from build123d import *

# Parameters (mm, degrees)
BOSS_EXTRUDE1_DEPTH = 63.5
SKETCH3_W           = 52.197
SKETCH3_H           = 52.197
BOSS_EXTRUDE2_DEPTH = 20.574
SKETCH_D_R          = 9.525
BOSS_EXTRUDE3_DEPTH = 38.1
CUT_EXTRUDE1_DEPTH  = 35.56
FILLET1_R           = 6.35
FILLET2_R           = 1.27
KEYWAY_START        = 6.8326
KEYWAY_DEPTH        = 51.3174
CHAMFER1_SIZE       = 0.381
SKETCH7_R           = 9.525
CUT_EXTRUDE3_DEPTH  = 123.174


with BuildPart() as part:
    # L,M → Boss-Extrude1 (new body)
    with BuildSketch(Plane.XY):
        Polygon((-66.675, 53.975), (66.675, 53.975), (66.675, 151.07969491), (52.451, 165.30369491), (52.451, 212.64830509), (18.97330509, 246.126), (-18.97330509, 246.126), (-52.451, 212.64830509), (-52.451, 165.30369491), (-66.675, 151.07969491), align=None)
    extrude(amount=BOSS_EXTRUDE1_DEPTH)

    # Sketch3 → Boss-Extrude2 (add)
    with BuildSketch(Plane.XY.offset(63.5)):
        with Locations((0, 188.976)):
            Rectangle(SKETCH3_W, SKETCH3_H)
    extrude(amount=BOSS_EXTRUDE2_DEPTH)

    # D → Boss-Extrude3 (add)
    with BuildSketch(Plane.XY.offset(84.074)):
        with Locations((0, 188.976)):
            Circle(SKETCH_D_R)
    extrude(amount=BOSS_EXTRUDE3_DEPTH)

    # Sketch5 → Cut-Extrude1 (cut)
    with BuildSketch(Plane.XY.offset(63.5)):
        Polygon((66.675, 87.45269491), (33.19730509, 53.975), (66.675, 53.975), align=None)
        Polygon((-66.675, 53.975), (-66.675, 87.45269491), (-33.19730509, 53.975), align=None)
    extrude(amount=-CUT_EXTRUDE1_DEPTH, mode=Mode.SUBTRACT)

    # Fillet1
    fillet1_edges = [part.edges().sort_by_distance(p)[0] for p in [
        (-26.0985, 215.0745, 73.787),
        (-26.0985, 162.8775, 73.787),
        (26.0985, 162.8775, 73.787),
        (26.0985, 215.0745, 73.787),
    ]]
    fillet(fillet1_edges, radius=FILLET1_R)

    # Fillet2
    fillet2_edges = [part.edges().sort_by_distance(p)[0] for p in [
        (66.675, 119.26619491, 63.5),
        (49.936152545, 70.713847455, 63.5),
        (59.563, 158.19169491, 63.5),
        (52.451, 188.976, 63.5),
        (35.712152545, 229.387152545, 63.5),
        (0, 53.975, 63.5),
        (0, 246.126, 63.5),
        (-35.712152545, 229.387152545, 63.5),
        (-52.451, 188.976, 63.5),
        (-59.563, 158.19169491, 63.5),
        (-66.675, 119.26619491, 63.5),
        (-49.936152545, 70.713847455, 63.5),
        (0, 162.8775, 63.5),
        (-26.0985, 188.976, 63.5),
        (26.0985, 188.976, 63.5),
        (0, 215.0745, 63.5),
        (-24.238628061, 164.737371939, 63.5),
        (24.238628061, 164.737371939, 63.5),
        (-24.238628061, 213.214628061, 63.5),
        (24.238628061, 213.214628061, 63.5),
    ]]
    fillet(fillet2_edges, radius=FILLET2_R)

    # Sketch6 → Keyway (cut, through all)
    with BuildSketch(Plane(origin=(0, 188.976, 0), x_dir=(-1, 0, 0), z_dir=(0, 1, 0)).offset(KEYWAY_START)):
        with BuildLine():
            Line((2.3876, 122.174), (2.3876, 89.154))
            ThreePointArc((2.3876, 89.154), (0, 86.7664), (-2.3876, 89.154))
            Line((-2.3876, 89.154), (-2.3876, 122.174))
            ThreePointArc((-2.3876, 122.174), (0, 124.5616), (2.3876, 122.174))
        make_face()
    extrude(amount=KEYWAY_DEPTH, mode=Mode.SUBTRACT)

    # Chamfer1
    chamfer1_edges = [part.edges().sort_by_distance(p)[0] for p in [
        (-5.830254497, 181.443818543, 122.174),
    ]]
    chamfer(chamfer1_edges, length=CHAMFER1_SIZE)

    # Sketch7 → Cut-Extrude3 (cut, through all)
    with BuildSketch(Plane(origin=(0, 0, 0), x_dir=(-1, 0, 0), z_dir=(0, 0, -1))):
        with Locations((0, 107.95)):
            Circle(SKETCH7_R)
    extrude(amount=-CUT_EXTRUDE3_DEPTH, mode=Mode.SUBTRACT)


solid = part.part
Can you work these out from the model? Positions are in its coordinate system, mm. A direction names the side the tool comes from. Give positions to 0.01 mm unless a question says otherwise; leave off trailing zeros. Order: outer loops, then holes, each group sorted by start corner. A loop starts at its lowest first (then second) coordinate and runs counter-clockwise, first axis right, second up. Notation, with made-up numbers: M 76.25,57 L 133.25,57 A24 ccw 133.25,69 Z; hole C 33,-21 d6. An arc over 180 degrees is marked long. One line per question, with ' | ' between items.
Item 1: Suppose I cut it at C-C, the plane z = 72.5. Write out the boundary of the cut face in (x, y).
Answer block:
outline: M -26.1,169.23 A6.35 ccw -19.75,162.88 L 19.75,162.88 A6.35 ccw 26.1,169.23 L 26.1,208.72 A6.35 ccw 19.75,215.07 L -19.75,215.07 A6.35 ccw -26.1,208.72 Z
Item 2: Suppose I cut it at B-B, the plane x = 0. Write out the boundary of the cut face in (y, z) (1 decimal).
Answer block:
outline: M 54,0 L 98.4,0 L 98.4,63.5 L 55.2,63.5 A1.3 ccw 54,62.2 Z; M 117.5,0 L 246.1,0 L 246.1,62.2 A1.3 ccw 244.9,63.5 L 216.3,63.5 A1.3 cw 215.1,64.8 L 215.1,84.1 L 198.5,84.1 L 198.5,86.8 L 195.8,86.8 L 195.8,122.2 L 179.8,122.2 L 179.5,121.8 L 179.5,84.1 L 162.9,84.1 L 162.9,64.8 A1.3 cw 161.6,63.5 L 117.5,63.5 Z
Item 3: We'd pull the mould along X, two halves only. Please class faces 1 (the face through (50.17, 70.95, 45.33)), 2 (the face through (0, 195.809, 105)), 3 (the face through (-59.209, 158.005, 63.138)): released by +X, released by -X, zero draft, split by the parting line, or undercut.
Answer block:
face 1: released by +X | face 2: undercut | face 3: released by -X
Item 4: Please list where these lines run through material, in increasing order: L1, parallel to Y at x = 0, z = 14 (3 decimals); L2, parallel to X at y = 107, z = 37 (1 decimal); L3, parallel to Z at x = 43, y = 122.
Answer block:
L1: y = 53.975 to 98.425, 117.475 to 246.126 | L2: x = -66.7 to -9.5, 9.5 to 66.7 | L3: z = 0 to 63.5
Item 5: For faces 4 (the face through (-26.098, 189, 74)), 5 (the face through (-50.17, 70.95, 45.33)), 6 (the face through (24.29, 213.16, 74.56)), 7 (the face through (4.4, 180.53, 102.67)), which set-ups out of +Z, -Z, +X, -X, +Y, -Y let a thin tool reach every point of the face, with its end or its side?
Answer block:
face 4: +Z, -X, +Y, -Y | face 5: +Z, -X, -Y | face 6: +Z, +X, +Y | face 7: +Z
Item 6: Suppose I cut it at A-A, the plane y = 107.95. Write out the boundary of the cut face in (x, z) (3 decimals).
Answer block:
outline: M -66.675,0 L -9.525,0 L -9.525,63.5 L -65.405,63.5 A1.27 ccw -66.675,62.23 Z; M 9.525,0 L 66.675,0 L 66.675,62.23 A1.27 ccw 65.405,63.5 L 9.525,63.5 Z
Item 7: I'm going to push flat-ended pins straight in: pin 1 Ø21 at (x, z) = (-9.5, 77) entering from -Y; pin 2 Ø2.5 at (y, z) = (196.5, 107.5) entering from +X; pin 3 Ø2 at (y, z) = (197.5, 79.5) entering from +X. Where does each tip first touch, or does it pass through?
Answer block:
pin 1: stops at y = 162.88 | pin 2: stops at x = 7.17 | pin 3: stops at x = 26.1
Item 8: Suppose I cut it at D-D, the plane z = 56. Write out the boundary of the cut face in (x, y) (3 decimals).
Answer block:
outline: M -66.675,87.453 L -33.197,53.975 L 33.197,53.975 L 66.675,87.453 L 66.675,151.08 L 52.451,165.304 L 52.451,212.648 L 18.973,246.126 L -18.973,246.126 L -52.451,212.648 L -52.451,165.304 L -66.675,151.08 Z; hole C 0,107.95 d19.05
